Build history of the part. All positions in model axes, mm. A direction names the side the tool comes from. Round coordinates to 2 decimals unless told otherwise and drop trailing zeros. Order: outer loops, then holes, each group sorted by start corner. A loop starts at its lowest first (then second) coordinate and runs counter-clockwise, first axis right, second up. Notation, with made-up numbers: (-22.5, 51.5) -> (33.5, 51.5) arc R22 cw to (33.5, 70.5) -> close; hole circle Ø9 at (13.25, 64.5). An arc over 180 degrees is marked (long way). Answer as a JSON object with one key per item and string values.
from build123d import *

# Parameters (mm, degrees)
CYLINDER010_R            = 2.1
CYLINDER010_DEPTH        = 43
CYLINDER011_R            = 4
CYLINDER011_DEPTH        = 12
CYLINDER012_R            = 2.3
CYLINDER012_DEPTH        = 71
CUBE018_W                = 7.4
CUBE018_H                = 3.2
CUBE018_DEPTH            = 12
CUBE019_W                = 7.4
CUBE019_H                = 3.52
CUBE019_DEPTH            = 12
PRISM011_DEPTH           = 34
PRISM011_PLACEMENT_ANGLE = 15
PRISM012_DEPTH           = 34
PRISM012_PLACEMENT_ANGLE = 75
PRISM013_DEPTH           = 21
CUBE017_W                = 14
CUBE017_H                = 23
CUBE017_DEPTH            = 34.2
CUBE016_W                = 13.8
CUBE016_H                = 23
CUBE016_DEPTH            = 12
PRISM009_DEPTH           = 23
PRISM009_ROLL_ANGLE      = 90
PRISM009_PITCH_ANGLE     = -14.999996
PRISM010_DEPTH           = 23
PRISM010_ROLL_ANGLE      = -90
PRISM010_PITCH_ANGLE     = -14.999996
PRISM010_PLACEMENT_ANGLE = -180
CUBE015_W                = 20
CUBE015_H                = 23
CUBE015_DEPTH            = 40


with BuildPart() as cylinder010:
    # cylinder010 → cylinder010 (new body)
    with BuildSketch(Plane.XY.offset(44.5)):
        Circle(CYLINDER010_R)
    extrude(amount=CYLINDER010_DEPTH)


with BuildPart() as cylinder011:
    # cylinder011 → cylinder011 (new body)
    with BuildSketch(Plane.XY.offset(34)):
        Circle(CYLINDER011_R)
    extrude(amount=CYLINDER011_DEPTH)


with BuildPart() as cylinder012:
    # cylinder012 → cylinder012 (new body)
    with BuildSketch(Plane(origin=(0, 35.5, 40), x_dir=(1, 0, 0), z_dir=(0, -1, 0))):
        Circle(CYLINDER012_R)
    extrude(amount=CYLINDER012_DEPTH)


with BuildPart() as cube018:
    # cube018 → cube018 (new body)
    with BuildSketch(Plane(origin=(-3.7, -8.5, 34), x_dir=(1, 0, 0), z_dir=(0, 0, 1))):
        with Locations((3.7, 1.6)):
            Rectangle(CUBE018_W, CUBE018_H)
    extrude(amount=CUBE018_DEPTH)


with BuildPart() as cube019:
    # cube019 → cube019 (new body)
    with BuildSketch(Plane(origin=(-3.7, 5.14, 34), x_dir=(1, 0, 0), z_dir=(0, 0, 1))):
        with Locations((3.7, 1.76)):
            Rectangle(CUBE019_W, CUBE019_H)
    extrude(amount=CUBE019_DEPTH)


with BuildPart() as prism011:
    # prism011 → prism011 (new body)
    with BuildSketch(Plane.XY):
        Polygon((3, 0), (-1.5, 2.598076), (-1.5, -2.598076), align=None)
    extrude(amount=PRISM011_DEPTH)


with BuildPart() as prism011_1:
    # prism011 placement: moved
    add(prism011.part.moved(Location((7, 11.5, 49))).rotate(Axis((7, 11.5, 49), (0, 0, 1)), PRISM011_PLACEMENT_ANGLE))


with BuildPart() as prism012:
    # prism012 → prism012 (new body)
    with BuildSketch(Plane.XY):
        Polygon((3, 0), (-1.5, 2.598076), (-1.5, -2.598076), align=None)
    extrude(amount=PRISM012_DEPTH)


with BuildPart() as prism012_1:
    # prism012 placement: moved
    add(prism012.part.moved(Location((-7, 11.5, 49))).rotate(Axis((-7, 11.5, 49), (0, 0, -1)), PRISM012_PLACEMENT_ANGLE))


with BuildPart() as prism013:
    # prism013 → prism013 (new body)
    with BuildSketch(Plane(origin=(-10.5, 0, 76), x_dir=(0, 1, 0), z_dir=(1, 0, 0))):
        Polygon((3.1, 0), (1.55, 2.684679), (-1.55, 2.684679), (-3.1, 0), (-1.55, -2.684679), (1.55, -2.684679), align=None)
    extrude(amount=PRISM013_DEPTH)


with BuildPart() as group007:
    # cube017 → cube017 (new body)
    with BuildSketch(Plane(origin=(-7, -11.5, 48.9), x_dir=(1, 0, 0), z_dir=(0, 0, 1))):
        with Locations((7, 11.5)):
            Rectangle(CUBE017_W, CUBE017_H)
    extrude(amount=CUBE017_DEPTH)

    # Group007: union cylinder010, cylinder011, cylinder012, cube018, cube019, prism011, prism012, prism013
    add(cylinder010.part)
    add(cylinder011.part)
    add(cylinder012.part)
    add(cube018.part)
    add(cube019.part)
    add(prism011_1.part)
    add(prism012_1.part)
    add(prism013.part)


with BuildPart() as cube016:
    # cube016 → cube016 (new body)
    with BuildSketch(Plane(origin=(-6.9, -11.5, 34), x_dir=(1, 0, 0), z_dir=(0, 0, 1))):
        with Locations((6.9, 11.5)):
            Rectangle(CUBE016_W, CUBE016_H)
    extrude(amount=CUBE016_DEPTH)


with BuildPart() as prism009:
    # prism009 → prism009 (new body)
    with BuildSketch(Plane.XY):
        Polygon((3, 0), (-1.5, 2.598076), (-1.5, -2.598076), align=None)
    extrude(amount=PRISM009_DEPTH)


with BuildPart() as prism009_1:
    # prism009 roll: moved
    add(prism009.part.rotate(Axis((0, 0, 0), (1, 0, 0)), PRISM009_ROLL_ANGLE))


with BuildPart() as prism009_2:
    # prism009 pitch: moved
    add(prism009_1.part.rotate(Axis((0, 0, 0), (0, 1, 0)), PRISM009_PITCH_ANGLE))


with BuildPart() as prism009_3:
    # prism009 placement: moved
    add(prism009_2.part.moved(Location((7, 11.500001, 45.35))))


with BuildPart() as prism010:
    # prism010 → prism010 (new body)
    with BuildSketch(Plane.XY):
        Polygon((3, 0), (-1.5, 2.598076), (-1.5, -2.598076), align=None)
    extrude(amount=PRISM010_DEPTH)


with BuildPart() as prism010_1:
    # prism010 roll: moved
    add(prism010.part.rotate(Axis((0, 0, 0), (1, 0, 0)), PRISM010_ROLL_ANGLE))


with BuildPart() as prism010_2:
    # prism010 pitch: moved
    add(prism010_1.part.rotate(Axis((0, 0, 0), (0, 1, 0)), PRISM010_PITCH_ANGLE))


with BuildPart() as prism010_3:
    # prism010 placement: moved
    add(prism010_2.part.moved(Location((-7, 11.500001, 45.35))).rotate(Axis((-7, 11.500001, 45.35), (0, 0, 1)), PRISM010_PLACEMENT_ANGLE))


with BuildPart() as side_slider:
    # cube015 → cube015 (new body)
    with BuildSketch(Plane(origin=(-10, -11.5, 46), x_dir=(1, 0, 0), z_dir=(0, 0, 1))):
        with Locations((10, 11.5)):
            Rectangle(CUBE015_W, CUBE015_H)
    extrude(amount=CUBE015_DEPTH)

    # Group006: union cube016, prism009, prism010
    add(cube016.part)
    add(prism009_3.part)
    add(prism010_3.part)

    # difference004: cut Group007
    add(group007.part, mode=Mode.SUBTRACT)


solid = side_slider.part
1) Probe L1, parallel to Z at x = 0, y = 4.25; L2, parallel to X at y = 0, z = 84.1; L3, parallel to Z at x = -1.25, y = 3.5. List the from-to ranges inside material, lowest first. Write a range as from..to.
Checked values:
{"L1": "z = 34..37.7, 42.3..48.9, 83.1..86", "L2": "x = -10..-2.1, 2.1..10", "L3": "z = 46..48.9, 83.1..86"}
2) Cut at B-B, the plane y = 0. Count the separate pieces of the cut face and the enclosed holes in it, plus the area to 3 significant figures.
Checked values:
{"separate pieces": "4", "enclosed holes": "0", "area": "342 mm²"}
3) Cut at A-A, the plane z = 40. Give the cut face in (x, y).
Checked values:
{"outline": "(-6.9, -11.5) -> (-2.3, -11.5) -> (-2.3, -8.5) -> (-3.7, -8.5) -> (-3.7, -5.3) -> (-2.3, -5.3) -> (-2.3, -3.27) arc R4 cw to (-2.3, 3.27) -> (-2.3, 5.14) -> (-3.7, 5.14) -> (-3.7, 8.66) -> (-2.3, 8.66) -> (-2.3, 11.5) -> (-6.9, 11.5) -> close; (2.3, -11.5) -> (6.9, -11.5) -> (6.9, 11.5) -> (2.3, 11.5) -> (2.3, 8.66) -> (3.7, 8.66) -> (3.7, 5.14) -> (2.3, 5.14) -> (2.3, 3.27) arc R4 cw to (2.3, -3.27) -> (2.3, -5.3) -> (3.7, -5.3) -> (3.7, -8.5) -> (2.3, -8.5) -> close"}
4) Pull direction Z, two halves, no side cores. Call faces 1 (the face through (8, 0, 73.315)), 2 (the face through (8.479, -2.314, 77.361)), 3 (the face through (2.003, 0.631, 47.43)), 4 (the face through (-2.4, 0.2, 86)): pulls with the +Z half, pulls with the -Z half, needs draft (parallel to the pull), parting line crosses it, or undercut.
Checked values:
{"face 1": "undercut", "face 2": "undercut", "face 3": "needs draft", "face 4": "pulls with the +Z half"}
5) Flat gauge pins, fed straight in: pin 1 Ø3.5 at (y, z) = (1.5, 39) entering from -X; pin 2 Ø3.5 at (x, y) = (9, 0.5) entering from -Z; pin 3 Ø3.5 at (y, z) = (-7.5, 40.5) entering from +X. Where does each tip first touch, or does it go through?
Checked values:
{"pin 1": "stops at x = -6.9", "pin 2": "stops at z = 43.48", "pin 3": "stops at x = 6.9"}
6) Which spindle directions (+Z, -Z, +X, -X, +Y, -Y) get a long thin tool onto all of the face, cutting with end or side? Do faces 5 (the face through (7, -3, 66)), 6 (the face through (8.046, 10.424, 65.762)), 7 (the face through (3.7, 7, 40)), 8 (the face through (-9, 0, 73.315)), 9 (the face through (-6.9, 0, 39)). Say none if no direction does.
Checked values:
{"face 5": "+Y, -Y", "face 6": "+Y", "face 7": "-Z", "face 8": "+X, -X", "face 9": "-Z, -X, +Y, -Y"}
7) Cut at D-D, the plane z = 50.5. Give the cut face in (x, y), plus the area to 4 significant figures.
Checked values:
{"outline": "(-10, -11.5) -> (-7, -11.5) -> (-7, 9.38) -> (-9.12, 11.5) -> (-10, 11.5) -> close; (7, -11.5) -> (10, -11.5) -> (10, 11.5) -> (9.12, 11.5) -> (7, 9.38) -> close", "area": "133.5 mm²"}
8) Cut at C-C, the plane y = 7.25. Give the cut face in (x, z), plus the area to 3 significant figures.
Checked values:
{"outline": "(-10, 46) -> (-9.77, 46) -> (-6.9, 43.13) -> (-6.9, 34) -> (-3.7, 34) -> (-3.7, 46) -> (3.7, 46) -> (3.7, 34) -> (6.9, 34) -> (6.9, 43.13) -> (9.77, 46) -> (10, 46) -> (10, 86) -> (-10, 86) -> close; hole (-7, 48.9) -> (7, 48.9) -> (7, 83.1) -> (-7, 83.1) -> close", "area": "406 mm²"}
